```python
from build123d import *

# Parameters (mm, degrees)
SKIZZE1_W                       = 5
SKIZZE1_H                       = 80
SKIZZE1_W_2                     = 50
SKIZZE1_H_2                     = 5
SKIZZE2_W                       = 20
SKIZZE2_H                       = 10
AUFSATZ_LINEAR_AUSTRAGEN1_DEPTH = 30
SKIZZE3_R                       = 5
SCHNITT_LINEAR_AUSTRAGEN1_DEPTH = 30


with BuildPart() as part:
    # Skizze1 → Rotation1 (revolve)
    with BuildSketch(Plane.XY, mode=Mode.PRIVATE) as rotation1_sk:
        with Locations((-2.5, 40)):
            Rectangle(SKIZZE1_W, SKIZZE1_H)
        with Locations((25, 72.5)):
            Rectangle(SKIZZE1_W_2, SKIZZE1_H_2)
    revolve(rotation1_sk.sketch.rotate(Axis((0, 0, 0), (1, 0, 0)), 90), axis=Axis((0, 0, 0), (1, 0, 0)))

    # Skizze2 → Aufsatz-Linear austragen1 (add)
    with BuildSketch(Plane(origin=(0, 0, 0), x_dir=(0, 0, -1), z_dir=(1, 0, 0))):
        Rectangle(SKIZZE2_W, SKIZZE2_H)
    extrude(amount=AUFSATZ_LINEAR_AUSTRAGEN1_DEPTH)

    # Skizze3 → Schnitt-Linear austragen1 (cut)
    with BuildSketch(Plane.XZ.offset(5)):
        with Locations(Location((20, 0, 0), (0, 0, 270))):
            Circle(SKIZZE3_R)
    extrude(amount=-SCHNITT_LINEAR_AUSTRAGEN1_DEPTH, mode=Mode.SUBTRACT)


solid = part.part
```
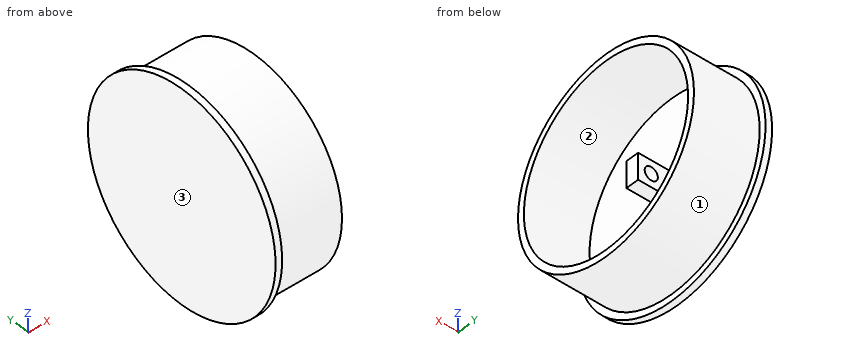
Build history of the part. All positions in model axes, mm. Face numbers are marked on the shaded views. Give positions to 0.01 mm unless a question says otherwise; leave off trailing zeros. Loops run counter-clockwise (first coordinate to the right, second up) from the corner with the lowest first, then second, coordinate; pieces in that order, holes last. Notation, with made-up numbers: (3, -0.5) - (7, -0.5) arc R25 cw to (7, 27.5) - close; hole circle Ø2 at (71, -18.5). An arc over 180 degrees is marked (long way). Use a Markdown table: item, result.
(1) Drop flat-ended pins along their axis: pin 1 Ø16 at (x, z) = (11, 2.5) entering from +Y; pin 2 Ø10 at (x, z) = (10.5, -31.5) entering from +Y; pin 3 Ø3 at (x, z) = (30, -58) entering from -Y. Give the stop position or say it passes through.
Taken from the geometry:
| item | result |
|---|---|
| pin 1 | y = 75 |
| pin 2 | y = 70.16 |
| pin 3 | y = -49.32 |
(2) Wall check: line 1 along Y through (x, z) = (12, 0); line 2 along Y through (x, z) = (25, -4); line 3 along X through (y, z) = (0, 0). Give the ranges that are in metal, low to high.
Taken from the geometry:
| item | result |
|---|---|
| line 1 | -75 to -70, -5 to 5, 70 to 75 |
| line 2 | -74.89 to -69.89, -5 to 5, 69.89 to 74.89 |
| line 3 | -5 to 15, 25 to 30 |
(3) Band-saw the part on C-C (x = 6.5). Give the cut face in (y, z), and give its area (3 significant figures).
Taken from the geometry:
| item | result |
|---|---|
| outline | circle Ø150 at (0, 0); (-5, -10) - (5, -10) - (5, 10) - (-5, 10) - close; hole circle Ø140 at (0, 0) |
| area | 2,480 mm2 |
(4) Band-saw the part on D-D (y = 0). Give the cut face in (x, z).
Taken from the geometry:
| item | result |
|---|---|
| outline | (-5, -80) - (0, -80) - (0, -75) - (50, -75) - (50, -70) - (0, -70) - (0, -10) - (30, -10) - (30, 10) - (0, 10) - (0, 70) - (50, 70) - (50, 75) - (0, 75) - (0, 80) - (-5, 80) - close; hole circle Ø10 at (20, 0) |
(5) Band-saw the part on B-B (z = 0). Give the cut face in (x, y).
Taken from the geometry:
| item | result |
|---|---|
| outline | (-5, -80) - (0, -80) - (0, -75) - (50, -75) - (50, -70) - (0, -70) - (0, -5) - (15, -5) - (15, 5) - (0, 5) - (0, 70) - (50, 70) - (50, 75) - (0, 75) - (0, 80) - (-5, 80) - close; (25, -5) - (30, -5) - (30, 5) - (25, 5) - close |
(6) Pull direction Y, two halves, no side cores. Call the marked faces 1, 2 and 3: +Y half, -Y half, draft (parallel to the pull), parting line (faces both ways), or undercut.
Taken from the geometry:
| item | result |
|---|---|
| face 1 | parting line |
| face 2 | undercut |
| face 3 | draft |
(7) Band-saw the part on A-A (x = 20). Give the cut face in (y, z), and give its area (3 significant figures).
Taken from the geometry:
| item | result |
|---|---|
| outline | circle Ø150 at (0, 0); (-5, -10) - (5, -10) - (5, -5) - (-5, -5) - close; (-5, 5) - (5, 5) - (5, 10) - (-5, 10) - close; hole circle Ø140 at (0, 0) |
| area | 2,380 mm2 |
